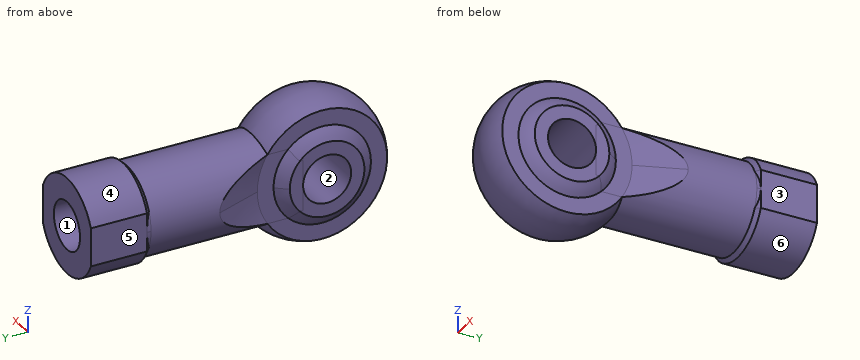
```python
from build123d import *

# Parameters (mm, degrees)
F9_R          = 3
F10_DEPTH     = 27
F11_DEPTH     = 7.5
F12_DEPTH     = 13.5
F13_T2_ANGLE  = 157.4663491
F13_T6_DEPTH  = 3.6837572556
F13_S7_R      = 5.5
F13_T8_DEPTH  = 3
F13_T12_DEPTH = 3.6837572556
F13_S13_R     = 5.5
F13_T14_DEPTH = 3
F13_T16_ANGLE = 157.4663491
F13_T20_DEPTH = 3.6837572556
F13_S21_R     = 5.5
F13_T22_DEPTH = 3
F13_T26_DEPTH = 3.6837572556
F13_S27_R     = 5.5
F13_T28_DEPTH = 3


# Not quite as in the source:
# - a fillet or chamfer that OpenCascade refuses, or shapes differently, is made with other operations: its cross-section is extruded or revolved along the edge and cut away or added


with BuildPart() as f7:
    # F6 (on Top) → F7 (revolve)
    with BuildSketch(Plane.XY):
        with BuildLine():
            Line((-4.5, 4.65), (-4.5, 3))
            Line((-4.5, 3), (4.5, 3))
            Line((4.5, 3), (4.5, 4.65))
            ThreePointArc((4.5, 4.65), (4.0013141648, 5.4121962233), (3.375, 6.073529129))
            ThreePointArc((3.375, 6.073529129), (0, 7.35), (-3.375, 6.073529129))
            ThreePointArc((-3.375, 6.073529129), (-4.0013141648, 5.4121962233), (-4.5, 4.65))
        make_face()
        with BuildLine():
            Line((-3.375, 8.0956714755), (-3.375, 6.073529129))
            ThreePointArc((-3.375, 6.073529129), (0, 7.35), (3.375, 6.073529129))
            Line((3.375, 6.073529129), (3.375, 8.0956714755))
            ThreePointArc((3.375, 8.0956714755), (0, 9), (-3.375, 8.0956714755))
        make_face()
    revolve(axis=Axis((0, 0, 0), (1, 0, 0)))

    # F9 (on offset) → F10 (join)
    with BuildSketch(Plane.XZ.offset(-30)):
        with BuildLine():
            ThreePointArc((-5.5, 0), (0, -5.5), (5.5, 0))
            ThreePointArc((5.5, 0), (0, 5.5), (-5.5, 0))
        make_face()
        Circle(F9_R, mode=Mode.SUBTRACT)
        Circle(F9_R)
    extrude(amount=F10_DEPTH)

    # F9 (on offset) → F11 (join)
    with BuildSketch(Plane.XZ.offset(-30)):
        with BuildLine():
            ThreePointArc((-5.5, 0), (0, 5.5), (5.5, 0))
            Line((5.5, 0), (5.5, 2.3979157617))
            ThreePointArc((5.5, 2.3979157617), (0, 6), (-5.5, 2.3979157617))
            Line((-5.5, 2.3979157617), (-5.5, 0))
        make_face()
        with BuildLine():
            Line((5.5, -2.3979157617), (5.5, 0))
            ThreePointArc((5.5, 0), (0, -5.5), (-5.5, 0))
            Line((-5.5, 0), (-5.5, -2.3979157617))
            ThreePointArc((-5.5, -2.3979157617), (0, -6), (5.5, -2.3979157617))
        make_face()
    extrude(amount=F11_DEPTH)

    # F9 (on offset) → F12 (cut)
    with BuildSketch(Plane.XZ.offset(-30)):
        Circle(F9_R)
    extrude(amount=F12_DEPTH, mode=Mode.SUBTRACT)

    # F13: chamfer of 0.5 on 6 edges, made by hand

    # F13_s1 → F13_t2 (revolve, cut)
    with BuildSketch(Plane(origin=(0, 0, 0), x_dir=(0, 1, 0), z_dir=(0.1953783305, 0, -0.980727948))):
        Polygon((22.5, 5.5), (23, 6), (22.5, 6), align=None)
    revolve(axis=Axis((0, 22.5, 0), (0, -1, 0)), revolution_arc=F13_T2_ANGLE, mode=Mode.SUBTRACT)


with BuildPart() as f13_tool4:
    # F13_s5 → F13_t6 (new body)
    with BuildSketch(Plane.XY):
        Polygon((5, 22.5), (5.5, 23), (5.5, 22.5), align=None)
    extrude(amount=F13_T6_DEPTH)

    # F13_s7 → F13_t8 (cut, symmetric)
    with BuildSketch(Plane.XZ.offset(-22.8)):
        Circle(F13_S7_R)
    extrude(amount=F13_T8_DEPTH, both=True, mode=Mode.SUBTRACT)


with BuildPart() as f7_1:
    add(f7.part)

    # F13_t3: cut F13_tool4
    add(f13_tool4.part, mode=Mode.SUBTRACT)


with BuildPart() as f13_tool10:
    # F13_s11 → F13_t12 (new body)
    with BuildSketch(Plane.XY.offset(3.6837572556)):
        Polygon((-5, 22.5), (-5.5, 23), (-5.5, 22.5), align=None)
    extrude(amount=-F13_T12_DEPTH)

    # F13_s13 → F13_t14 (cut, symmetric)
    with BuildSketch(Plane.XZ.offset(-22.8)):
        Circle(F13_S13_R)
    extrude(amount=F13_T14_DEPTH, both=True, mode=Mode.SUBTRACT)


with BuildPart() as f7_2:
    add(f7_1.part)

    # F13_t9: cut F13_tool10
    add(f13_tool10.part, mode=Mode.SUBTRACT)

    # F13_s15 → F13_t16 (revolve, cut)
    with BuildSketch(Plane(origin=(0, 0, 0), x_dir=(0, 1, 0), z_dir=(-0.1953783305, 0, 0.980727948))):
        Polygon((22.5, 5.5), (23, 6), (22.5, 6), align=None)
    revolve(axis=Axis((0, 22.5, 0), (0, -1, 0)), revolution_arc=F13_T16_ANGLE, mode=Mode.SUBTRACT)


with BuildPart() as f13_tool18:
    # F13_s19 → F13_t20 (new body)
    with BuildSketch(Plane.XY.offset(-3.6837572556)):
        Polygon((5, 22.5), (5.5, 23), (5.5, 22.5), align=None)
    extrude(amount=F13_T20_DEPTH)

    # F13_s21 → F13_t22 (cut, symmetric)
    with BuildSketch(Plane.XZ.offset(-22.8)):
        Circle(F13_S21_R)
    extrude(amount=F13_T22_DEPTH, both=True, mode=Mode.SUBTRACT)


with BuildPart() as f7_3:
    add(f7_2.part)

    # F13_t17: cut F13_tool18
    add(f13_tool18.part, mode=Mode.SUBTRACT)


with BuildPart() as f13_tool24:
    # F13_s25 → F13_t26 (new body)
    with BuildSketch(Plane.XY):
        Polygon((-5, 22.5), (-5.5, 23), (-5.5, 22.5), align=None)
    extrude(amount=-F13_T26_DEPTH)

    # F13_s27 → F13_t28 (cut, symmetric)
    with BuildSketch(Plane.XZ.offset(-22.8)):
        Circle(F13_S27_R)
    extrude(amount=F13_T28_DEPTH, both=True, mode=Mode.SUBTRACT)


with BuildPart() as f7_4:
    add(f7_3.part)

    # F13_t23: cut F13_tool24
    add(f13_tool24.part, mode=Mode.SUBTRACT)

    # F6 (on Top) → F14 (revolve, cut)
    with BuildSketch(Plane.XY):
        with BuildLine():
            Line((4.5, 4.65), (4.5, 3))
            Line((4.5, 3), (6.5, 3))
            Line((6.5, 3), (6.5, 16.6815384113))
            Line((6.5, 16.6815384113), (3.375, 8.0956714755))
            Line((3.375, 8.0956714755), (3.375, 6.073529129))
            ThreePointArc((3.375, 6.073529129), (4.0013141648, 5.4121962233), (4.5, 4.65))
        make_face()
        with BuildLine():
            Line((-6.5, 3), (-4.5, 3))
            Line((-4.5, 3), (-4.5, 4.65))
            ThreePointArc((-4.5, 4.65), (-4.0013141648, 5.4121962233), (-3.375, 6.073529129))
            Line((-3.375, 6.073529129), (-3.375, 8.0956714755))
            Line((-3.375, 8.0956714755), (-6.5, 16.6815384113))
            Line((-6.5, 16.6815384113), (-6.5, 3))
        make_face()
    revolve(axis=Axis((0, 0, 0), (1, 0, 0)), mode=Mode.SUBTRACT)


solid = f7_4.part
```
Here's how the part is built. I have some questions about the finished solid (model axes, mm). Face numbers are marked on the shaded views. A direction names the side the tool comes from. Give positions to 0.01 mm unless a question says otherwise; leave off trailing zeros. Loops run counter-clockwise (first coordinate to the right, second up) from the corner with the lowest first, then second, coordinate; pieces in that order, holes last. Notation, with made-up numbers: M -24.75,-3 L -19.75,-3 A18 ccw -19.75,21 Z; hole C -21.75,31 d3. An arc over 180 degrees is marked long. Put each result on its own line as item: value. Start each with the question number.
(1) I want a section at A-A on y = 22. Please give me the cut outline in (x, z), then the cut area to 3 significant figures.
(2) I need wall thicknesses on line 1 along Z through (x, y) = (0, 21.75); line 2 along Z through (x, y) = (-1.25, 0); line 3 along X through (y, z) = (0, 7) (3 decimals). Which ranges of each line are inside material? Lowest first, please. Write a range as [from, to].
(3) For the marked faces 4, 5 and 6, which set-ups out of +Z, -Z, +X, -X, +Y, -Y let a thin tool reach every point of the face, with its end or its side?
(4) If we mould it in two halves opening along X, with no side actions, what happens to the marked faces 1, 2 and 3? For each: +X half, -X half, draft (parallel to the pull), parting line (faces both ways), or undercut.
(5) Will these pins go through, and if not, where does the flat tip stop? pin 1 Ø5.5 at (y, z) = (0, 0) entering from +X; pin 2 Ø0.5 at (y, z) = (3.5, 0.5) entering from -X; pin 3 Ø5 at (x, z) = (0, 0) entering from +Y; pin 4 Ø1 at (x, z) = (-0.5, -3.5) entering from -Y.
Answer block:
1. outline: C 0,0 d11; hole C 0,0 d6
1. area: 66.8 mm^2
2. line 1: [-5.5, -3], [3, 5.5]
2. line 2: [-8.88, -3], [3, 8.88]
2. line 3: [-3.375, 3.375]
3. face 4: +Z, +Y
3. face 5: +Z, -Z, -X, +Y, -Y
3. face 6: -Z, +Y
4. face 1: undercut
4. face 2: draft
4. face 3: +X half
5. pin 1: through
5. pin 2: x = -4.5
5. pin 3: y = 16.5
5. pin 4: y = -8.47
